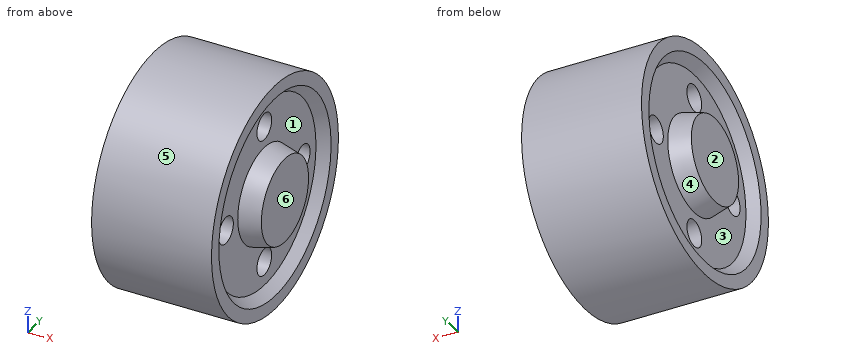
from build123d import *

# Parameters (mm, degrees)
SKETCH2_R          = 5
CUT_EXTRUDE2_DEPTH = 50


with BuildPart() as part:
    # Sketch1 → Revolve1 (revolve)
    with BuildSketch(Plane.XY, mode=Mode.PRIVATE) as revolve1_sk:
        Polygon((0, 0), (0, 16), (7.745966692, 18), (7.745966692, 35), (3.745966692, 38), (3.745966692, 43), (48.745966692, 43), (48.745966692, 38), (44.745966692, 35), (44.745966692, 18), (52.491933385, 16), (52.491933385, 0), align=None)
    revolve(revolve1_sk.sketch.rotate(Axis((0, 0, 0), (1, 0, 0)), 180), axis=Axis((0, 0, 0), (1, 0, 0)))

    # Sketch2 → Cut-Extrude2 (cut)
    with BuildSketch(Plane(origin=(52.491933385, 0, 0), x_dir=(0, 0, -1), z_dir=(1, 0, 0))):
        with Locations(Location((0, 26, 0), (0, 0, 90))):
            Circle(SKETCH2_R)
        with Locations(Location((26, 0, 0), (0, 0, 90))):
            Circle(SKETCH2_R)
        with Locations(Location((0, -26, 0), (0, 0, 90))):
            Circle(SKETCH2_R)
        with Locations(Location((-26, 0, 0), (0, 0, 90))):
            Circle(SKETCH2_R)
    extrude(amount=-CUT_EXTRUDE2_DEPTH, mode=Mode.SUBTRACT)


solid = part.part
Could you check a few things on this model? Use its own coordinates, in mm. Face numbers are marked on the shaded views. A direction names the side the tool comes from. Round coordinates to 2 decimals unless told otherwise and drop trailing zeros. Write each loop counter-clockwise with the first axis right and the second up, starting at its lowest first coordinate (ties: lowest second). Pieces come first, ordered by that corner, then holes. Notation, with made-up numbers: (-21, 51.25) - (-1, 51.25) arc R17 cw to (-1, 83.25) - close; hole circle Ø6 at (-13.5, 44). An arc over 180 degrees is marked (long way). Use a Markdown table: item, result.
Q1. I want a section at A-A (y = 0). List the corners of the cut face in (x, z) for me.
Output values:
| item | result |
|---|---|
| outline | (0, -16) - (7.75, -18) - (7.75, -21) - (44.75, -21) - (44.75, -18) - (52.49, -16) - (52.49, 16) - (44.75, 18) - (44.75, 21) - (7.75, 21) - (7.75, 18) - (0, 16) - close; (3.75, -43) - (48.75, -43) - (48.75, -38) - (44.75, -35) - (44.75, -31) - (7.75, -31) - (7.75, -35) - (3.75, -38) - close; (3.75, 38) - (7.75, 35) - (7.75, 31) - (44.75, 31) - (44.75, 35) - (48.75, 38) - (48.75, 43) - (3.75, 43) - close |
Q2. For pin 1 (4 mm diameter, centred on x = 23.5, y = 11.5, fed in from -Z); pin 2 (6 mm diameter, centred on y = -26, z = 0, fed in from +X); pin 3 (1 mm diameter, centred on x = 9.5, z = -6.5, fed in from -Y); pin 4 (1.5 mm diameter, centred on x = 7.5, z = 15.5, fed in from +Y), each with a flat end and sliding along its axis, tell me the tip position at first contact or that it passes through.
Output values:
| item | result |
|---|---|
| pin 1 | z = -41.94 |
| pin 2 | through |
| pin 3 | y = -42.58 |
| pin 4 | y = 40.39 |
Q3. For the marked faces 1, 2 and 3, which set-ups out of +Z, -Z, +X, -X, +Y, -Y let a thin tool reach every point of the face, with its end or its side?
Output values:
| item | result |
|---|---|
| face 1 | +X |
| face 2 | +Z, -Z, -X, +Y, -Y |
| face 3 | -X |
Q4. Thinking about a two-plate mould opening in Z: for the marked faces 4, 5 and 6, which applies, released by +Z, released by -Z, zero draft, split by the parting line, or undercut?
Output values:
| item | result |
|---|---|
| face 4 | undercut |
| face 5 | split by the parting line |
| face 6 | zero draft |
Q5. I want a section at D-D (x = 6). List the corners of the cut face in (y, z) for me, plus the area to 3 significant figures.
Output values:
| item | result |
|---|---|
| outline | circle Ø86 at (0, 0); circle Ø35.1 at (0, 0); hole circle Ø72.62 at (0, 0) |
| area | 2,630 mm2 |
Q6. I want a section at C-C (x = 38). List the corners of the cut face in (y, z) for me.
Output values:
| item | result |
|---|---|
| outline | circle Ø86 at (0, 0); hole circle Ø10 at (-26, 0); hole circle Ø10 at (0, -26); hole circle Ø10 at (0, 26); hole circle Ø10 at (26, 0) |
Q7. Please list where these lines run through material, in increasing order: L1, parallel to Z at x = 35, y = 0; L2, parallel to X at y = 33, z = 9; L3, parallel to Z at x = 38, y = -28.
Output values:
| item | result |
|---|---|
| L1 | -43 to -31, -21 to 21, 31 to 43 |
| L2 | 7.75 to 44.75 |
| L3 | -32.63 to -4.58, 4.58 to 32.63 |
